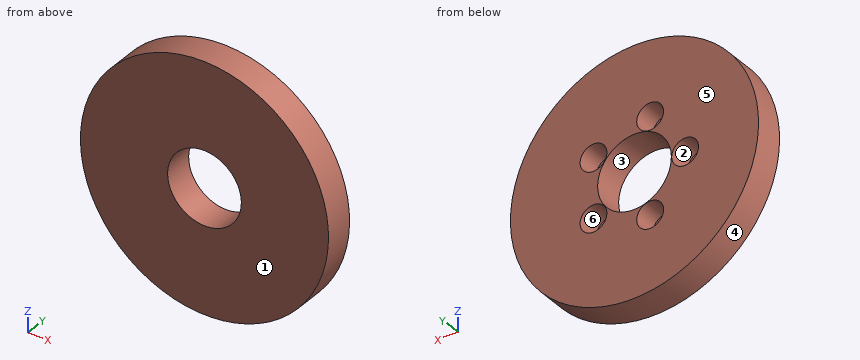
from build123d import *

# Parameters (mm, degrees)
SKETCH1_R             = 92.5
BOSS_EXTRUDE1_DEPTH   = 22
SKETCH2_R             = 27.5
CUT_EXTRUDE1_DEPTH    = 133.651799837
SKETCH3_R             = 10
CUT_EXTRUDE2_DEPTH    = 16.88371
CIRPATTERN1_START     = 5.11628988
CIRPATTERN1_OUTLINE_R = 10
CIRPATTERN1_DEPTH     = 16.88371012


# Read off the part's stored shape, not the designer's step: CirPattern1
with BuildPart() as part:
    # Sketch1 → Boss-Extrude1 (new body)
    with BuildSketch(Plane(origin=(0, 0, 0), x_dir=(1, 0, 0), z_dir=(0, 1, 0))):
        with Locations(Location((0, 0, 0), (0, 0, 270))):
            Circle(SKETCH1_R)
    extrude(amount=BOSS_EXTRUDE1_DEPTH)

    # Sketch2 → Cut-Extrude1 (cut, through all)
    with BuildSketch(Plane(origin=(0, 0, 0), x_dir=(1, 0, 0), z_dir=(0, 1, 0))):
        with Locations(Location((0, 0, 0), (0, 0, 270))):
            Circle(SKETCH2_R)
    extrude(amount=CUT_EXTRUDE1_DEPTH, mode=Mode.SUBTRACT)

    # Sketch3 → Cut-Extrude2 (cut)
    with BuildSketch(Plane(origin=(0, 22, 0), x_dir=(1, 0, 0), z_dir=(0, 1, 0))):
        with Locations(Location((-37.756047361, 0, 0), (0, 0, 270))):
            Circle(SKETCH3_R)
    extrude(amount=-CUT_EXTRUDE2_DEPTH, mode=Mode.SUBTRACT)

    # CirPattern1 outline → CirPattern1 (cut)
    with BuildSketch(Plane(origin=(0, 0, 0), x_dir=(1, 0, 0), z_dir=(0, 1, 0)).offset(CIRPATTERN1_START)):
        with Locations((-11.667260275, -35.908134872)):
            Circle(CIRPATTERN1_OUTLINE_R)
        with Locations((30.545283955, -22.192447823)):
            Circle(CIRPATTERN1_OUTLINE_R)
        with Locations((30.545283955, 22.192447823)):
            Circle(CIRPATTERN1_OUTLINE_R)
        with Locations((-11.667260275, 35.908134872)):
            Circle(CIRPATTERN1_OUTLINE_R)
    extrude(amount=CIRPATTERN1_DEPTH, mode=Mode.SUBTRACT)


solid = part.part
CAD build for the part. Positions are in the model's coordinates, mm. Face numbers are marked on the shaded views. A direction names the side the tool comes from. Give positions to 0.01 mm unless a question says otherwise; leave off trailing zeros. Order: outer loops, then holes, each group sorted by start corner. A loop starts at its lowest first (then second) coordinate and runs counter-clockwise, first axis right, second up. Notation, with made-up numbers: (-1, -5) - (26, -5) arc R16 ccw to (26, 18) - close; hole circle Ø5 at (19, -26.75). An arc over 180 degrees is marked (long way). Answer in a Markdown table with one row per item.
1. Pull direction Z, two halves, no side cores. Call the marked faces 1, 2, 3 and 4: pulls with the +Z half, pulls with the -Z half, needs draft (parallel to the pull), parting line crosses it, or undercut.
Data:
| item | result |
|---|---|
| face 1 | needs draft |
| face 2 | undercut |
| face 3 | undercut |
| face 4 | parting line crosses it |
2. Saw through at A-A, the plane z = 0. Give the cut face in (x, y), plus the area to 3 significant figures.
Data:
| item | result |
|---|---|
| outline | (-92.5, 0) - (-27.5, 0) - (-27.5, 22) - (-27.76, 22) - (-27.76, 5.12) - (-47.76, 5.12) - (-47.76, 22) - (-92.5, 22) - close; (27.5, 0) - (92.5, 0) - (92.5, 22) - (27.5, 22) - close |
| area | 2,520 mm² |
3. Saw through at D-D, the plane z = -74. Give the cut face in (x, y), plus the area to 3 significant figures.
Data:
| item | result |
|---|---|
| outline | (-55.5, 0) - (55.5, 0) - (55.5, 22) - (-55.5, 22) - close |
| area | 2,440 mm² |
4. Saw through at B-B, the plane y = 3. Give the cut face in (x, z).
Data:
| item | result |
|---|---|
| outline | circle Ø185 at (0, 0); hole circle Ø55 at (0, 0) |
5. Tool access for the marked faces 5 and 6: list every direction of +Z, -Z, +X, -X, +Y, -Y with a clear straight run to the whole face (end or side of a thin tool).
Data:
| item | result |
|---|---|
| face 5 | +Z, -Z, +X, -X, +Y |
| face 6 | +Y |
6. Flat gauge pins, fed straight in: pin 1 (6 mm diameter, centred on y = 3.5, z = 60.5, fed in from -X); pin 2 (6 mm diameter, centred on x = 26, z = -27, fed in from +Y); pin 3 (22 mm diameter, centred on x = -37, z = -3.5, fed in from +Y); pin 4 (10 mm diameter, centred on x = 10, y = 8, fed in from -Z). Where does each tip first touch, or does it go through?
Data:
| item | result |
|---|---|
| pin 1 | stops at x = -72.46 |
| pin 2 | stops at y = 5.12 |
| pin 3 | stops at y = 22 |
| pin 4 | stops at z = -92.36 |
7. Saw through at C-C, the plane y = 16.5. Give the cut face in (x, z), plus the area to 3 significant figures.
Data:
| item | result |
|---|---|
| outline | circle Ø185 at (0, 0); hole circle Ø20 at (-37.76, 0); hole circle Ø55 at (0, 0); hole circle Ø20 at (-11.67, -35.91); hole circle Ø20 at (-11.67, 35.91); hole circle Ø20 at (30.55, -22.19); hole circle Ø20 at (30.55, 22.19) |
| area | 22,900 mm² |
8. Probe probe 1 along X at (y, z) = (12, 0); probe 2 along X at (y, z) = (10.25, 37); probe 3 along Z at (x, y) = (14.5, 3.75). List the from-to ranges inside material, lowest first. Write a range as [from, to].
Data:
| item | result |
|---|---|
| probe 1 | x = [-92.5, -47.76], [-27.76, -27.5], [27.5, 92.5] |
| probe 2 | x = [-84.78, -21.61], [-1.73, 84.78] |
| probe 3 | z = [-91.36, -23.37], [23.37, 91.36] |
